```python
from build123d import *

# Parameters (mm, degrees)
SKETCH_R        = 4.05
SKETCH_W        = 19.9
SKETCH_H        = 6.4
PAD_DEPTH       = 10
SKETCH002_W     = 3
SKETCH002_H     = 6.9
POCKET001_DEPTH = 12
SKETCH003_R     = 2.25
POCKET_DEPTH    = 6
SKETCH004_R     = 2.25
POCKET002_DEPTH = 25.901


with BuildPart() as part:
    # Sketch → Pad (new body)
    with BuildSketch(Plane.XY):
        with BuildLine():
            ThreePointArc((12.95, 0), (0, 12.95), (-12.95, 0))
            Line((-12.95, 0), (-12.95, -30.2))
            Line((-12.95, -30.2), (12.95, -30.2))
            Line((12.95, -30.2), (12.95, 0))
        make_face()
        Circle(SKETCH_R, mode=Mode.SUBTRACT)
        with Locations((0, -25)):
            Rectangle(SKETCH_W, SKETCH_H, mode=Mode.SUBTRACT)
    extrude(amount=PAD_DEPTH)

    # Sketch002 → Pocket001 (cut)
    with BuildSketch(Plane.XY.offset(10)):
        with Locations((-8.5, 0)):
            Rectangle(SKETCH002_W, SKETCH002_H)
    extrude(amount=-POCKET001_DEPTH, mode=Mode.SUBTRACT)

    # Sketch003 → Pocket (cut, symmetric)
    with BuildSketch(Plane.YZ.offset(-9.95)):
        with Locations((0, 5)):
            Circle(SKETCH003_R)
    extrude(amount=POCKET_DEPTH, both=True, mode=Mode.SUBTRACT)

    # Sketch004 → Pocket002 (cut, through all)
    with BuildSketch(Plane.YZ.offset(12.95)):
        with Locations((0, 5)):
            Circle(SKETCH004_R)
    extrude(amount=-POCKET002_DEPTH, mode=Mode.SUBTRACT)


solid = part.part
```
Geometry check sheet. Reference: the model listing, model coordinates, mm. A direction names the side the tool comes from. Give positions to 0.01 mm unless a question says otherwise; leave off trailing zeros. Write each loop counter-clockwise with the first axis right and the second up, starting at its lowest first coordinate (ties: lowest second). Pieces come first, ordered by that corner, then holes.
1) Gauge pin test, flat ends, axial feed: pin 1 (3.5 mm diameter, centred on y = 0, z = 5, fed in from +X); pin 2 (2 mm diameter, centred on x = -3.5, z = 3.5, fed in from +Y); pin 3 (6 mm diameter, centred on x = -8, z = 7, fed in from +Y); pin 4 (2 mm diameter, centred on x = 9, z = 6.5, fed in from +Y). Record the tip position at first contact, or that the pin passes through.
2) Section check B-B, the plane z = 5. Record the boundary of the cut face in (x, y), and give its area (3 significant figures).
3) Material ranges on L1, parallel to Y at x = 0, z = 4.25; L2, parallel to X at y = -24, z = 4.5; L3, parallel to Y at x = -4.75, z = 3.75, recorded low to high.
4) Release check for a two-part mould opening along Z. For faces 3 (the flat face through (0, -8, 0)), 4 (the cylindrical face through (-5.158, 2.146, 5.676)), 5 (the cylindrical face through (-11.45, -0.29, 7.23)), 6 (the flat face through (0, -28.2, 5)) record: pulls with the +Z half, pulls with the -Z half, needs draft (parallel to the pull), parting line crosses it, or undercut.
5) Access from +Z, -Z, +X, -X, +Y, -Y to the whole of each face (thin tool, end or side, straight path). Record for faces 1 (the flat face through (12.95, -15, 5)), 2 (the flat face through (-9, 3.45, 5)).
6) Section check A-A, the plane x = 0. Record the boundary of the cut face in (y, z), and give its area (4 significant figures).
7) Section check D-D, the plane x = 7.25. Record the boundary of the cut face in (y, z), and give its area (3 significant figures).
8) Section check C-C, the plane y = -25.5. Record the boundary of the cut face in (x, z).
Computed:
1. pin 1: passes through
1. pin 2: stops at y = 12.71
1. pin 3: stops at y = 11.95
1. pin 4: stops at y = 10.18
2. outline: (-12.95, -30.2) - (12.95, -30.2) - (12.95, -2.25) - (3.37, -2.25) arc R4.05 cw to (-3.37, -2.25) - (-7, -2.25) - (-7, -3.45) - (-10, -3.45) - (-10, -2.25) - (-12.95, -2.25) - close; (-12.75, 2.25) - (-10, 2.25) - (-10, 3.45) - (-7, 3.45) - (-7, 2.25) - (-3.37, 2.25) arc R4.05 cw to (3.37, 2.25) - (12.75, 2.25) arc R12.95 ccw to start; hole (-9.95, -28.2) - (9.95, -28.2) - (9.95, -21.8) - (-9.95, -21.8) - close
2. area: 778 mm2
3. L1: y = -30.2 to -28.2, -21.8 to -4.05, 4.05 to 12.95
3. L2: x = -12.95 to -9.95, 9.95 to 12.95
3. L3: y = -30.2 to -28.2, -21.8 to -1.87, 1.87 to 12.05
4. face 3: pulls with the -Z half
4. face 4: undercut
4. face 5: undercut
4. face 6: needs draft
5. face 1: +Z, -Z, +X, +Y, -Y
5. face 2: +Z, -Z
6. outline: (-30.2, 0) - (-28.2, 0) - (-28.2, 10) - (-30.2, 10) - close; (-21.8, 0) - (-4.05, 0) - (-4.05, 10) - (-21.8, 10) - close; (4.05, 0) - (12.95, 0) - (12.95, 10) - (4.05, 10) - close
6. area: 286.5 mm2
7. outline: (-30.2, 0) - (-28.2, 0) - (-28.2, 10) - (-30.2, 10) - close; (-21.8, 0) - (10.73, 0) - (10.73, 10) - (-21.8, 10) - close; hole circle Ø4.5 at (0, 5)
7. area: 329 mm2
8. outline: (-12.95, 0) - (-9.95, 0) - (-9.95, 10) - (-12.95, 10) - close; (9.95, 0) - (12.95, 0) - (12.95, 10) - (9.95, 10) - close
